Could you check a few things on this model? Use its own coordinates, in mm. Face numbers are marked on the shaded views. Give positions to 0.01 mm unless a question says otherwise; leave off trailing zeros. Write each loop counter-clockwise with the first axis right and the second up, starting at its lowest first coordinate (ties: lowest second). Pieces come first, ordered by that corner, then holes. Notation, with made-up numbers: (-29, 51) - (4, 51) arc R23 cw to (4, 65) - close; hole circle Ø4 at (85, 3). An arc over 180 degrees is marked (long way). Write item = value, one per line.
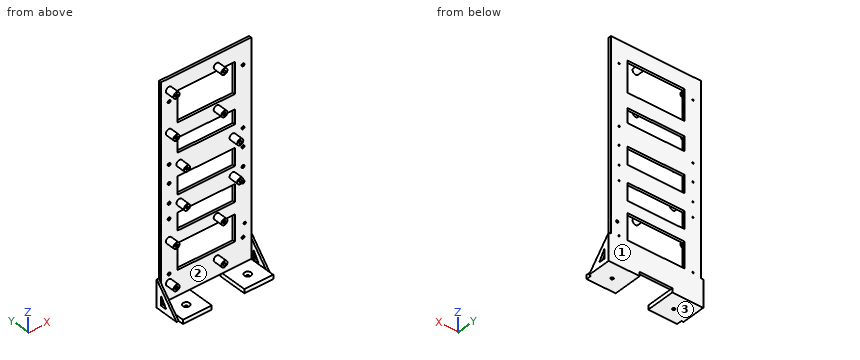
from build123d import *

# Parameters (mm, degrees)
SKETCH_R            = 1.4
SKETCH_W            = 69.6
SKETCH_H            = 21.261902
SKETCH_H_2          = 37.270492
SKETCH_H_3          = 17.445648
SKETCH_H_4          = 21.010353
SKETCH_H_5          = 31.498865
PAD_DEPTH           = 3
SKETCH001_R         = 3.7
SKETCH001_R_2       = 1.5
PAD001_DEPTH        = 11
SKETCH002_W         = 35
SKETCH002_H         = 5
PAD002_DEPTH        = 32
PAD002_DEPTH_BACK   = 3
HOLE_D              = 3.4
HOLE_DEPTH          = 25
HOLE_CSINK_D        = 8
HOLE_CSINK_ANGLE    = 90
PAD003_DEPTH        = 2.5
HOLE002_D           = 1.71
HOLE002_DEPTH       = 25
HOLE002_CSINK_D     = 3.5
HOLE002_CSINK_ANGLE = 90


with BuildPart() as part:
    # Sketch → Pad (new body)
    with BuildSketch(Plane.XZ):
        Polygon((-54.8, 257.006653), (-54.8, 20.406653), (-54.8, 0), (54.8, 0), (54.8, 20.406653), (54.8, 257.006653), align=None)
        with Locations((46.99, 45.5)):
            Circle(SKETCH_R, mode=Mode.SUBTRACT)
        with Locations((0, 127.83873)):
            Rectangle(SKETCH_W, SKETCH_H, mode=Mode.SUBTRACT)
        with Locations((0, 219.541237)):
            Rectangle(SKETCH_W, SKETCH_H_2, mode=Mode.SUBTRACT)
        with Locations((0, 174.45137)):
            Rectangle(SKETCH_W, SKETCH_H_3, mode=Mode.SUBTRACT)
        with Locations((0, 85.985882)):
            Rectangle(SKETCH_W, SKETCH_H_4, mode=Mode.SUBTRACT)
        with Locations((0, 45.447963)):
            Rectangle(SKETCH_W, SKETCH_H_5, mode=Mode.SUBTRACT)
    extrude(amount=-PAD_DEPTH)

    # Sketch001 → Pad001 (join)
    with BuildSketch(Plane.XZ):
        with Locations((-45, 243.58207)):
            Circle(SKETCH001_R)
        with Locations((-45, 243.58207)):
            Circle(SKETCH001_R_2, mode=Mode.SUBTRACT)
        with Locations((13, 243.58207)):
            Circle(SKETCH001_R)
        with Locations((13, 243.58207)):
            Circle(SKETCH001_R_2, mode=Mode.SUBTRACT)
        with Locations((-45, 194.58207)):
            Circle(SKETCH001_R)
        with Locations((-45, 194.58207)):
            Circle(SKETCH001_R_2, mode=Mode.SUBTRACT)
        with Locations((13, 194.58207)):
            Circle(SKETCH001_R)
        with Locations((13, 194.58207)):
            Circle(SKETCH001_R_2, mode=Mode.SUBTRACT)
        with Locations((-45, 69.260145)):
            Circle(SKETCH001_R)
        with Locations((-45, 69.260145)):
            Circle(SKETCH001_R_2, mode=Mode.SUBTRACT)
        with Locations((-45, 20.260145)):
            Circle(SKETCH001_R)
        with Locations((-45, 20.260145)):
            Circle(SKETCH001_R_2, mode=Mode.SUBTRACT)
        with Locations((13, 20.260145)):
            Circle(SKETCH001_R)
        with Locations((13, 20.260145)):
            Circle(SKETCH001_R_2, mode=Mode.SUBTRACT)
        with Locations((13, 69.260145)):
            Circle(SKETCH001_R)
        with Locations((13, 69.260145)):
            Circle(SKETCH001_R_2, mode=Mode.SUBTRACT)
        with Locations((-32.25, 107.638794)):
            Circle(SKETCH001_R)
        with Locations((-32.25, 107.638794)):
            Circle(SKETCH001_R_2, mode=Mode.SUBTRACT)
        with Locations((32.25, 107.638794)):
            Circle(SKETCH001_R)
        with Locations((32.25, 107.638794)):
            Circle(SKETCH001_R_2, mode=Mode.SUBTRACT)
        with Locations((32.25, 152.638794)):
            Circle(SKETCH001_R)
        with Locations((32.25, 152.638794)):
            Circle(SKETCH001_R_2, mode=Mode.SUBTRACT)
        with Locations((-32.25, 152.638794)):
            Circle(SKETCH001_R)
        with Locations((-32.25, 152.638794)):
            Circle(SKETCH001_R_2, mode=Mode.SUBTRACT)
    extrude(amount=PAD001_DEPTH)

    # Sketch002 → Pad002 (join, two sides)
    with BuildSketch(Plane.XZ) as pad002_sk:
        with Locations((-37.3, -2.5)):
            Rectangle(SKETCH002_W, SKETCH002_H)
        with Locations((37.3, -2.5)):
            Rectangle(SKETCH002_W, SKETCH002_H)
    extrude(amount=PAD002_DEPTH)
    extrude(pad002_sk.sketch, amount=-PAD002_DEPTH_BACK)

    # Hole
    with Locations(Plane.XY):
        with Locations((-37.3, -16), (37.3, -16)):
            CounterSinkHole(HOLE_D / 2, HOLE_CSINK_D / 2, depth=HOLE_DEPTH, counter_sink_angle=HOLE_CSINK_ANGLE)

    # Sketch004 (on DatumPlane) → Pad003 (join)
    with BuildSketch(Plane.YZ.offset(54.8)):
        Polygon((-25.8, -5), (3, -5), (3, 28), align=None)
        Polygon((-10.8, 1), (-3, 13), (-3, 1), align=None, mode=Mode.SUBTRACT)
    pad003 = extrude(amount=PAD003_DEPTH)

    # Mirrored: Pad003 across YZ
    add(pad003.mirror(Plane.YZ))

    # Hole002
    with Locations(Plane.XZ):
        with Locations((44.8, 157), (-44.8, 135), (44.8, 135), (-44.8, 112), (-44.8, 94), (44.8, 112), (44.8, 94), (-44.8, 30), (44.8, 30), (-44.8, 157), (-44.8, 230), (44.8, 230)):
            CounterSinkHole(HOLE002_D / 2, HOLE002_CSINK_D / 2, depth=HOLE002_DEPTH, counter_sink_angle=HOLE002_CSINK_ANGLE)


with BuildPart() as part_1:
    # Body placement: moved
    add(part.part.moved(Location((0.2, -1, 0))))


solid = part_1.part
1. If we section it at C-C, the plane x = 4.5: Please give me the cut outline in (y, z), and give its area (3 significant figures).
Filled sheet:
outline = (-1, 0) - (2, 0) - (2, 29.7) - (-1, 29.7) - close; (-1, 61.2) - (2, 61.2) - (2, 75.48) - (-1, 75.48) - close; (-1, 96.49) - (2, 96.49) - (2, 117.21) - (-1, 117.21) - close; (-1, 138.47) - (2, 138.47) - (2, 165.73) - (-1, 165.73) - close; (-1, 183.17) - (2, 183.17) - (2, 200.91) - (-1, 200.91) - close; (-1, 238.18) - (2, 238.18) - (2, 257.01) - (-1, 257.01) - close
area = 386 mm2
2. Thinking about a two-plate mould opening in Z: for the marked faces 1, 2 and 3, which applies, pulls with the +Z half, pulls with the -Z half, needs draft (parallel to the pull), parting line crosses it, or undercut?
Filled sheet:
face_1 = needs draft
face_2 = undercut
face_3 = pulls with the -Z half
3. If we section it at B-B, the plane y = -7.5: Count the separate pieces of the cut face and the enclosed holes in it, and give its area (3 significant figures).
Filled sheet:
separate_pieces = 16
enclosed_holes = 12
area = 859 mm2
4. For pin 1 (2.5 mm diameter, centred on x = 32.45, z = 107.64, fed in from -Y); pin 2 (4 mm diameter, centred on x = -18, y = -28.5, fed in from -Z); pin 3 (1.5 mm diameter, centred on x = 8, y = 0, fed in from -Z); pin 4 (0.9 mm diameter, centred on y = 1, z = 48.5, fed in from -X), each with a flat end and sliding along its axis, tell me the tip position at first contact or that it passes through.
Filled sheet:
pin_1 = -1
pin_2 = -5
pin_3 = 0
pin_4 = -54.6
5. If we section it at A-A, the plane x = -23: Please give me the cut outline in (y, z).
Filled sheet:
outline = (-33, -5) - (2, -5) - (2, 29.7) - (-1, 29.7) - (-1, 0) - (-33, 0) - close; (-1, 61.2) - (2, 61.2) - (2, 75.48) - (-1, 75.48) - close; (-1, 96.49) - (2, 96.49) - (2, 117.21) - (-1, 117.21) - close; (-1, 138.47) - (2, 138.47) - (2, 165.73) - (-1, 165.73) - close; (-1, 183.17) - (2, 183.17) - (2, 200.91) - (-1, 200.91) - close; (-1, 238.18) - (2, 238.18) - (2, 257.01) - (-1, 257.01) - close
6. I need wall thicknesses on line 1 (Z direction, x = 19.5, y = -0.5); line 2 (Z direction, x = -32.05, y = -3); line 3 (X direction, y = 0.5, z = 230) (3 decimals). Which ranges of each line are inside material? Lowest first, please.
Filled sheet:
line_1 = 0 to 29.7, 61.2 to 75.48, 96.49 to 117.21, 138.47 to 165.73, 183.17 to 200.91, 238.18 to 257.01
line_2 = -5 to 0, 103.94 to 106.14, 109.14 to 111.34, 148.94 to 151.14, 154.14 to 156.34
line_3 = -54.6 to -45.455, -43.745 to -34.6, 35 to 44.145, 45.855 to 55
